```python
from build123d import *

# Parameters (mm, degrees)
F0_R     = 8.37382
F1_DEPTH = 3.81
F2_R     = 7.084201
F3_DEPTH = 20.32
F4_W     = 2.192053
F4_H     = 23.016576
F5_DEPTH = 0.254
F6_W     = 2.192054
F6_H     = 22.390274
F7_DEPTH = 0.254


with BuildPart() as f1:
    # F0 (on Top) → F1 (new body)
    with BuildSketch(Plane.XY):
        Circle(F0_R)
    extrude(amount=F1_DEPTH)

    # F2 (on face) → F3 (join)
    with BuildSketch(Plane.XY.offset(3.81)):
        Circle(F2_R)
    extrude(amount=F3_DEPTH)

    # F4 (on Right) → F5 (join)
    with BuildSketch(Plane.YZ):
        with Locations((5.166987, -11.508288)):
            Rectangle(F4_W, F4_H)
    extrude(amount=F5_DEPTH)

    # F6 (on Right) → F7 (join)
    with BuildSketch(Plane.YZ):
        with Locations((-4.540686, -11.195137)):
            Rectangle(F6_W, F6_H)
    extrude(amount=F7_DEPTH)


solid = f1.part
```
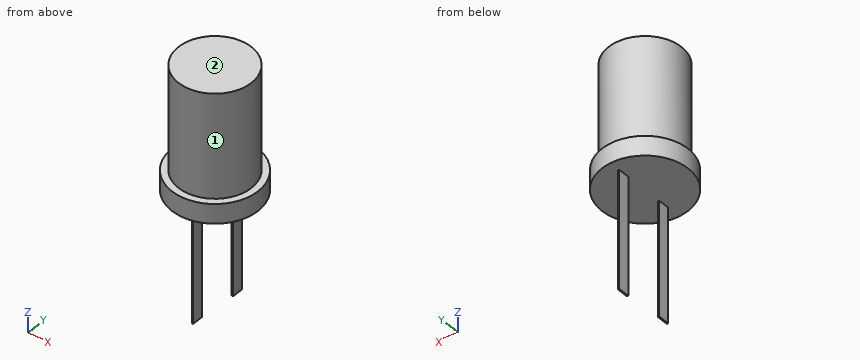
Verification items for the finished model (mm, model axes). Face numbers are marked on the shaded views. A direction names the side the tool comes from. Give positions to 0.01 mm unless a question says otherwise; leave off trailing zeros. Write each loop counter-clockwise with the first axis right and the second up, starting at its lowest first coordinate (ties: lowest second). Pieces come first, ordered by that corner, then holes. Notation, with made-up numbers: (45.5, -35.5) - (103.5, -35.5) arc R18 ccw to (103.5, -22.5) - close; hole circle Ø3 at (32, 9). An arc over 180 degrees is marked (long way). Put each result on its own line as item: value.
Q1. Section check D-D on z = 17.5. Record the cut outline in (x, y), and give its area (3 significant figures).
Result:
outline: circle Ø14.17 at (0, 0)
area: 158 mm2
Q2. Scan lines: probe 1 along Z at (x, y) = (-6, -1); probe 2 along X at (y, z) = (5.25, -13); probe 3 along Z at (x, y) = (7, -4). Record each from-to range of solid material in increasing order. Write a range as from..to.
Result:
probe 1: 0..24.13
probe 2: 0..0.25
probe 3: 0..3.81
Q3. Depth check by flat-ended pin: P1, Ø10, axis at x = 4, z = -13.5, coming from the +Y side; P2, Ø2, axis at x = 3, z = 4, coming from the -Y side; P3, Ø0.7, axis at y = -4.5, z = -6, coming from the +X side. Enter the tip coordinate at first touch or a pass-through.
Result:
P1: y = 6.26
P2: y = -8.13
P3: x = 0.25
Q4. Section check C-C on x = -2.25. Record the cut outline in (y, z).
Result:
outline: (-8.07, 0) - (8.07, 0) - (8.07, 3.81) - (6.72, 3.81) - (6.72, 24.13) - (-6.72, 24.13) - (-6.72, 3.81) - (-8.07, 3.81) - close
Q5. Section check B-B on y = 0. Record the cut outline in (x, z).
Result:
outline: (-8.37, 0) - (8.37, 0) - (8.37, 3.81) - (7.08, 3.81) - (7.08, 24.13) - (-7.08, 24.13) - (-7.08, 3.81) - (-8.37, 3.81) - close
Q6. Set-up check for the marked faces 1 and 2: record each of +Z, -Z, +X, -X, +Y, -Y from which the full face is reachable in a straight line by a thin tool's end or side.
Result:
face 1: +Z
face 2: +Z, +X, -X, +Y, -Y
Q7. Section check A-A on z = -3. Record the cut outline in (x, y), and give its area (3 significant figures).
Result:
outline: (0, -5.64) - (0.25, -5.64) - (0.25, -3.44) - (0, -3.44) - close; (0, 4.07) - (0.25, 4.07) - (0.25, 6.26) - (0, 6.26) - close
area: 1.11 mm2
